Job drawing, mm, ordinate dimensions from the low corner. One solid piece. Round coordinates to 2 decimals unless told otherwise and drop trailing zeros. Order: outer loops, then holes, each group sorted by start corner. A loop starts at its lowest first (then second) coordinate and runs counter-clockwise, first axis right, second up. Notation, with made-up numbers: (-24, 7.25) -> (25, 7.25) arc R23 ccw to (25, 46.25) -> close; hole circle Ø11 at (22.25, 78). An arc over 180 degrees is marked (long way). Answer as a JSON object with one key per item and string values. Group by question number.
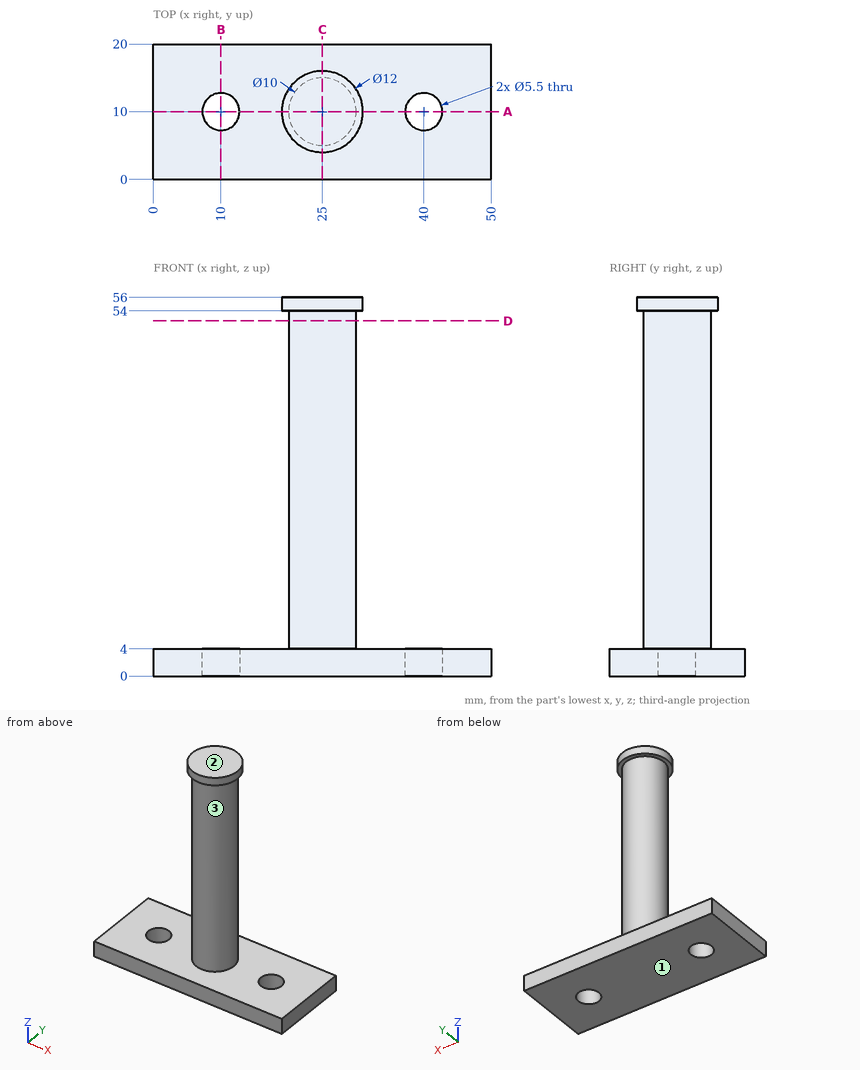
Q1. Drop flat-ended pins along their axis: pin 1 Ø1.5 at (x, y) = (45, 6.5) entering from +Z; pin 2 Ø1 at (y, z) = (16.5, 24) entering from -X; pin 3 Ø1.5 at (y, z) = (6.5, 20) entering from -X; pin 4 Ø5 at (x, y) = (26, 16.5) entering from -Z. Give the stop position or say it passes through.
Q2. Band-saw the part on A-A (y = 10). List the corners of the cut face in (x, z), plus the area to 3 significant figures.
Q3. Band-saw the part on B-B (x = 10). List the corners of the cut face in (y, z).
Q4. Band-saw the part on C-C (x = 25). List the corners of the cut face in (y, z), plus the area to 3 significant figures.
Q5. Wall check: line 1 (Y direction, x = 40, z = 1.1); line 2 (Z direction, x = 36.5, y = 12.25); line 3 (X direction, y = 12.75, z = 28). Give the ranges that are in metal, low to high. Write a range as [from, to].
Q6. Band-saw the part on D-D (z = 52.5). List the corners of the cut face in (x, y), plus the area to 3 significant figures.
Q7. Two-plate mould, pull along Z, no slides. Class the marked faces 1, 2 and 3: +Z half, -Z half, draft (parallel to the pull), parting line (faces both ways), or undercut.
Completed:
{
 "1": {"pin 1": "z = 4", "pin 2": "through", "pin 3": "x = 20.82", "pin 4": "z = 0"},
 "2": {"outline": "(0, 0) -> (7.25, 0) -> (7.25, 4) -> (0, 4) -> close; (12.75, 0) -> (37.25, 0) -> (37.25, 4) -> (30, 4) -> (30, 54) -> (31, 54) -> (31, 56) -> (19, 56) -> (19, 54) -> (20, 54) -> (20, 4) -> (12.75, 4) -> close; (42.75, 0) -> (50, 0) -> (50, 4) -> (42.75, 4) -> close", "area": "680 mm2"},
 "3": {"outline": "(0, 0) -> (7.25, 0) -> (7.25, 4) -> (0, 4) -> close; (12.75, 0) -> (20, 0) -> (20, 4) -> (12.75, 4) -> close"},
 "4": {"outline": "(0, 0) -> (20, 0) -> (20, 4) -> (15, 4) -> (15, 54) -> (16, 54) -> (16, 56) -> (4, 56) -> (4, 54) -> (5, 54) -> (5, 4) -> (0, 4) -> close", "area": "604 mm2"},
 "5": {"line 1": "[0, 7.25], [12.75, 20]", "line 2": "[0, 4]", "line 3": "[20.82, 29.18]"},
 "6": {"outline": "circle Ø10 at (25, 10)", "area": "78.5 mm2"},
 "7": {"face 1": "-Z half", "face 2": "+Z half", "face 3": "undercut"}
}
